```python
from build123d import *

# Parameters (mm, degrees)
F1_DEPTH = 80
F3_R     = 5


with BuildPart() as f1:
    # F0 (on Front) → F1 (new body)
    with BuildSketch(Plane.XZ):
        with BuildLine():
            Line((-52.3298562962, 0), (0, 0))
            Line((0, 0), (0, 2))
            Line((0, 2), (-52.3298562962, 2))
            ThreePointArc((-52.3298562962, 2), (-82.0233760889, 12.7436715119), (-97.9677842805, 40))
            Line((-97.9677842805, 40), (-100, 40))
            ThreePointArc((-100, 40), (-83.4443328334, 11.3247433143), (-52.3298562962, 0))
        make_face()
    extrude(amount=F1_DEPTH)

    # F2: F1 across face


with BuildPart() as f1_1:
    add(f1.part)
    add(f1.part.mirror(Plane(origin=(0, -40, 1), x_dir=(0, 1, 0), z_dir=(1, 0, 0))))

    # F3
    f3_edges = [f1_1.edges().sort_by_distance(p)[0] for p in [
        (-98.983892, -80, 40),
        (-98.983892, 0, 40),
        (98.983892, -80, 40),
        (98.983892, 0, 40),
    ]]
    fillet(f3_edges, radius=F3_R)


solid = f1_1.part
```
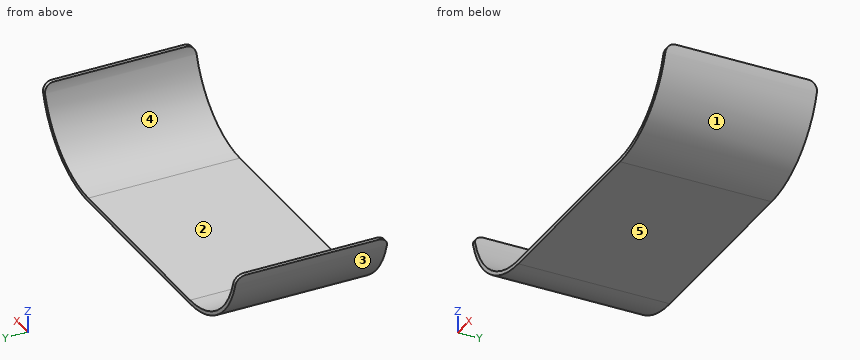
Here's how the part is built. I have some questions about the finished solid (model axes, mm). Face numbers are marked on the shaded views. A direction names the side the tool comes from. Coordinates: 2 decimals unless noted, no trailing zeros. Order: outer loops, then holes, each group sorted by start corner. A loop starts at its lowest first (then second) coordinate and runs counter-clockwise, first axis right, second up. Notation, with made-up numbers: (67.5, 45) - (108.5, 45) arc R15 ccw to (108.5, 57) - close; hole circle Ø8 at (61.25, 13.5). An arc over 180 degrees is marked (long way). One line per question, with ' | ' between items.
(1) Suppose I cut it at A-A on z = 37. List the corners of the cut face in (x, y) for me.
Report:
outline: (-99.37, -79.58) - (-97.31, -79.58) - (-97.31, -0.42) - (-99.37, -0.42) - close; (97.31, -79.58) - (99.37, -79.58) - (99.37, -0.42) - (97.31, -0.42) - close
(2) Will these pins go through, and if not, where does the flat tip stop? pin 1 (1 mm diameter, centred on y = -58, z = 29.5, fed in from +X); pin 2 (8 mm diameter, centred on y = -47.5, z = 8.5, fed in from +X); pin 3 (1 mm diameter, centred on x = 31.5, y = -16, fed in from +Z).
Report:
pin 1: stops at x = 97.1 | pin 2: stops at x = 84.79 | pin 3: stops at z = 2
(3) Suppose I cut it at D-D on z = 9. List the corners of the cut face in (x, y) for me, and give its area (3 significant figures).
Report:
outline: (-80.44, -80) - (-76.84, -80) - (-76.84, 0) - (-80.44, 0) - close; (76.84, -80) - (80.44, -80) - (80.44, 0) - (76.84, 0) - close | area: 577 mm2
(4) Suppose I cut it at C-C on x = 36. List the corners of the cut face in (y, z) for me.
Report:
outline: (-80, 0) - (0, 0) - (0, 2) - (-80, 2) - close
(5) Suppose I cut it at B-B on y = -8. List the corners of the cut face in (x, z) for me, and give its area (3 significant figures).
Report:
outline: (-100, 40) arc R48.41 ccw to (-52.33, 0) - (52.33, 0) arc R48.41 ccw to (100, 40) - (97.97, 40) arc R46.41 cw to (52.33, 2) - (-52.33, 2) arc R46.41 cw to (-97.97, 40) - close | area: 473 mm2
(6) If I drill on L1, parallel to Z at x = -16, y = -17.5; L2, parallel to X at y = -37, z = 20.5; L3, parallel to X at y = -56, z = 6, over which ranges is the centre line in solid material (lowest first)?
Report:
L1: z = 0 to 2 | L2: x = -91.88 to -89.41, 89.41 to 91.88 | L3: x = -75.67 to -71.18, 71.18 to 75.67
(7) If we mould it in two halves opening along X, with no side actions, what happens to the marked faces 3, 4 and 5? For each: pulls with the +X half, pulls with the -X half, needs draft (parallel to the pull), parting line crosses it, or undercut.
Report:
face 3: pulls with the -X half | face 4: undercut | face 5: needs draft
(8) For the marked faces 1 and 2, which set-ups out of +Z, -Z, +X, -X, +Y, -Y let a thin tool reach every point of the face, with its end or its side?
Report:
face 1: -Z, +X, +Y, -Y | face 2: +Z, +Y, -Y
